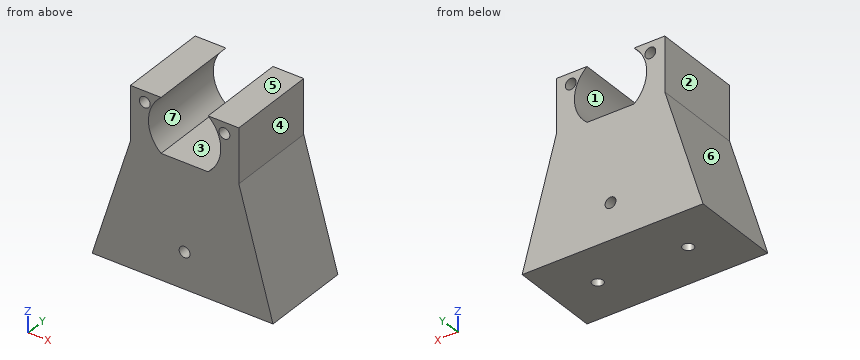
from build123d import *

# Parameters (mm, degrees)
F0_R     = 1.5
F1_DEPTH = 25
F2_R     = 1.5
F3_DEPTH = 10


with BuildPart() as f1:
    # F0 (on Front) → F1 (new body)
    with BuildSketch(Plane.XZ):
        with BuildLine():
            Line((6.5, 34), (15, 34))
            Line((15, 34), (15, 49))
            Line((15, 49), (6.5, 49))
            ThreePointArc((6.5, 49), (10, 41.5), (6.5, 34))
        make_face()
        with Locations((11, 46)):
            Circle(F0_R, mode=Mode.SUBTRACT)
        with BuildLine():
            Line((-15, 49), (-15, 34))
            Line((-15, 34), (-6.5, 34))
            ThreePointArc((-6.5, 34), (-10, 41.5), (-6.5, 49))
            Line((-6.5, 49), (-15, 49))
        make_face()
        with Locations((-11, 46)):
            Circle(F0_R, mode=Mode.SUBTRACT)
        Polygon((-15, 34), (-25.561607, 0), (24.438393, 0), (15, 34), (6.5, 34), (-6.5, 34), align=None)
        with Locations((0, 10)):
            Circle(F0_R, mode=Mode.SUBTRACT)
    extrude(amount=F1_DEPTH)

    # F2 (on face) → F3 (cut)
    with BuildSketch(Plane(origin=(0, 0, 0), x_dir=(1, 0, 0), z_dir=(0, 0, -1))):
        with Locations((-12.5, 12.5)):
            Circle(F2_R)
        with Locations((12.5, 12.5)):
            Circle(F2_R)
    extrude(amount=-F3_DEPTH, mode=Mode.SUBTRACT)


solid = f1.part
For this review, take the finished solid that the model builds, in its own axes (mm). Face numbers are marked on the shaded views. A direction names the side the tool comes from. Give positions to 0.01 mm unless a question says otherwise; leave off trailing zeros. Loops run counter-clockwise (first coordinate to the right, second up) from the corner with the lowest first, then second, coordinate; pieces in that order, holes last. Notation, with made-up numbers: M 2,20 L 12,20 A22 cw 12,45 Z; hole C -19,56.5 d11. An arc over 180 degrees is marked long. Put each result on its own line as item: value. Start each with the question number.
(1) Add section C-C, the plane z = 43. Write out the cut boundary in (x, y), then the cut area to 3 significant figures.
(2) For pin 1 (7.5 mm diameter, centred on y = -8, z = 45, fed in from -X); pin 2 (1.5 mm diameter, centred on x = -12.5, y = -12.5, fed in from -Z); pin 3 (1 mm diameter, centred on y = -3, z = 35.5, fed in from +X), all flat-tipped, find the tip position at first contact; note any pin that passes through.
(3) Add section B-B, the plane y = -15.5. Write out the cut boundary in (x, z).
(4) Wall thickness on L1, parallel to Y at x = -12.5, z = 3.75; L2, parallel to Z at x = 0, y = -17.75; L3, parallel to Z at x = 6, y = -4.25: over which ranges is each line inside the solid? List them lowest first.
(5) Add section A-A, the plane x = 0. Write out the cut boundary in (y, z).
(6) Add section D-D, the plane z = 6.5. Write out the cut boundary in (x, y), then the cut area to 3 significant figures.
(7) The part is to be moulded in two halves that separate along X. For the marked faces 5, 6 and 7, say which applies: +X half, -X half, draft (parallel to the pull), parting line (faces both ways), or undercut.
(8) Machinability: for the marked faces 1, 2, 3 and 4, which of the approach directions +Z, -Z, +X, -X, +Y, -Y give a long, thin tool a straight path to every point of the face, cutting with its end or side? Answer none if there is none.
Result:
1. outline: M -15,-25 L -9.88,-25 L -9.88,0 L -15,0 Z; M 9.88,-25 L 15,-25 L 15,0 L 9.88,0 Z
1. area: 256 mm^2
2. pin 1: stops at x = -15
2. pin 2: stops at z = 10
2. pin 3: stops at x = 15
3. outline: M -25.56,0 L 24.44,0 L 15,34 L 15,49 L 6.5,49 A9.79 cw 6.5,34 L -6.5,34 A9.79 cw -6.5,49 L -15,49 L -15,34 Z; hole C -11,46 d3; hole C 0,10 d3; hole C 11,46 d3
4. L1: y = -25 to -14, -11 to 0
4. L2: z = 0 to 8.5, 11.5 to 34
4. L3: z = 0 to 34
5. outline: M -25,0 L 0,0 L 0,8.5 L -25,8.5 Z; M -25,11.5 L 0,11.5 L 0,34 L -25,34 Z
6. outline: M -23.54,-25 L 22.63,-25 L 22.63,0 L -23.54,0 Z; hole C -12.5,-12.5 d3; hole C 12.5,-12.5 d3
6. area: 1,140 mm^2
7. face 5: draft
7. face 6: -X half
7. face 7: undercut
8. face 1: +Y, -Y
8. face 2: +Z, -X, +Y, -Y
8. face 3: +Z, +Y, -Y
8. face 4: +Z, +X, +Y, -Y
